Model file for the job. Use its own axes, mm. Face numbers are marked on the shaded views. A direction names the side the tool comes from. Round coordinates to 2 decimals unless told otherwise and drop trailing zeros. Write each loop counter-clockwise with the first axis right and the second up, starting at its lowest first coordinate (ties: lowest second). Pieces come first, ordered by that corner, then holes. Notation, with made-up numbers: (28, 82.25) - (87, 82.25) arc R29 ccw to (87, 117.25) - close; hole circle Ø7 at (-0.75, -9). An arc over 180 degrees is marked (long way). One line per item, written item: value.
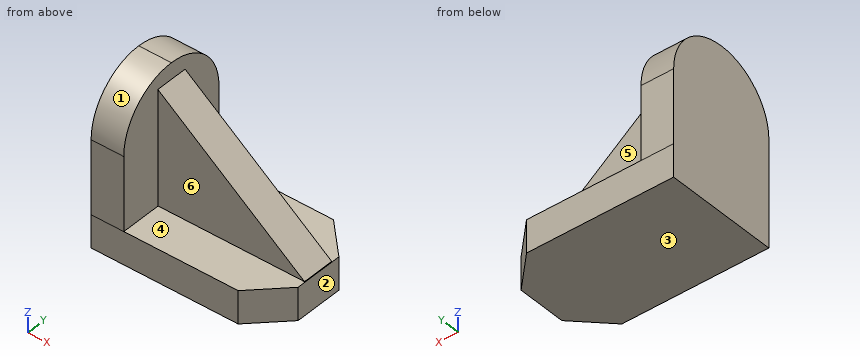
Autodesk Fusion 360 part; units mm, degrees
sketch "Horizontal" plane through (0, 0, 0) normal (0, 0, 1) x (1, 0, 0)
  line L0 (33, -21) -> (-33, -21)
  line L1 (-33, -21) -> (-33, 21)
  line L2 (-33, 21) -> (33, 21)
  line L3 (33, 21) -> (33, -21)
  line L4 (33, -21) -> (-33, 21) construction
  line L5 (-33, -21) -> (33, 21) construction
  dimension "d1" = 66
  dimension "d2" = 42
extrude "Extrude1" add sketch "Horizontal" along normal blind 12
chamfer "Chamfer1" distance 12 angle 45 2 edges at (33, -21, 6) (33, 21, 6)
sketch "Vertical" plane through (0, 0, 0) normal (0, 0, 1) x (1, 0, 0)
  line L0 (-33, 20.9715) -> (-21, 20.9715)
  line L1 (-21, 20.9715) -> (-21, -21.0285)
  line L2 (-21, -21.0285) -> (-33, -21.0285)
  line L3 (-33, -21.0285) -> (-33, 20.9715)
  line L4 (-33, 20.9715) -> (-21, 20.9715)
  line L5 (-21, 20.9715) -> (-21, -21.0285)
  line L6 (-21, -21.0285) -> (-33, -21.0285)
  line L7 (-33, -21.0285) -> (-33, 20.9715)
  line L8 (-33, -21) -> (-33, 21)
  dimension "d6" = 12
  dimension "d7" = 42
  dimension "d8" = 12
  dimension "d9" = 42
extrude "Extrude2" add sketch "Vertical" along normal blind 60 and the other way blind -12
fillet "Fillet1" radius 21 2 edges at (-27, -21.0285, 60) (-27, 20.9715, 60)
sketch "Triangle" plane through (0, 0, 0) normal (0, 1, 0) x (1, 0, 0)
  line L0 (-21.1404, -54.1172) -> (-21.1404, -12.1172)
  line L1 (-21.1404, -12.1172) -> (32.8596, -12.1172)
  line L2 (32.8596, -12.1172) -> (-21.1404, -54.1172)
  dimension "d16" = 42
  dimension "d17" = 54
extrude "Extrude3" add sketch "Triangle" along normal mid plane 12
equation "d17 = 66 mm - 12 mm"
1. Band-saw the part on C-C on y = -2. Write the cut outline in (x, z), plus the area to 4 significant figures.
Report:
outline: (-33, 0) - (33, 0) - (33, 12) - (-21, 12) - (-21, 12.12) - (32.86, 12.12) - (-21, 54.01) - (-21, 59.91) - (-33, 59.91) - close
area: 2,495 mm²
2. Band-saw the part on D-D on x = 15. Write the cut outline in (y, z), plus the area to 3 significant figures.
Report:
outline: (-21, 0) - (21, 0) - (21, 12) - (-21, 12) - close; (-6, 12.12) - (6, 12.12) - (6, 26.01) - (-6, 26.01) - close
area: 671 mm²
3. Band-saw the part on B-B on z = 8.5. Write the cut outline in (x, y).
Report:
outline: (-33, -21) - (21, -21) - (33, -9) - (33, 9) - (21, 21) - (-33, 21) - close
4. Drop flat-ended pins along their axis: pin 1 (5 mm diameter, centred on x = 7.5, y = -12.5, fed in from +Z); pin 2 (8 mm diameter, centred on y = -12, z = 26, fed in from +X); pin 3 (1.5 mm diameter, centred on y = -1.5, z = 53, fed in from +X). Give the stop position or say it passes through.
Report:
pin 1: z = 12
pin 2: x = -21
pin 3: x = -18.74
5. Mould opens along Z. For the marked faces 1, 2, 3 and 4 say: released by +Z, released by -Z, zero draft, split by the parting line, or undercut.
Report:
face 1: released by +Z
face 2: zero draft
face 3: released by -Z
face 4: undercut
6. Wall check: probe 1 along Y at (x, z) = (-28, 8); probe 2 along Y at (x, z) = (-2, 16.5); probe 3 along Z at (x, y) = (18, -9). Give the ranges that are in metal, low to high. Write a range as [from, to].
Report:
probe 1: [-21, 21]
probe 2: [-6, 6]
probe 3: [0, 12]
7. Tool access for the marked faces 5 and 6: list every direction of +Z, -Z, +X, -X, +Y, -Y with a clear straight run to the whole face (end or side of a thin tool).
Report:
face 5: +Z, +X, +Y
face 6: +Z, +X, -Y
8. Band-saw the part on A-A on x = -6. Write the cut outline in (y, z).
Report:
outline: (-21, 0) - (21, 0) - (21, 12) - (-21, 12) - close; (-6, 12.12) - (6, 12.12) - (6, 42.34) - (-6, 42.34) - close
